Can you work these out from the model? Positions are in its coordinate system, mm. Face numbers are marked on the shaded views. A direction names the side the tool comes from. Coordinates: 2 decimals unless noted, no trailing zeros. Loops run counter-clockwise (first coordinate to the right, second up) from the corner with the lowest first, then second, coordinate; pieces in that order, holes last. Notation, with made-up numbers: (79, 71) -> (135, 71) arc R32 cw to (135, 100) -> close; hole circle Ø3 at (-1, 6). An arc over 180 degrees is marked (long way). Put each result on its own line as item: value. Start each with the question number.
Item 1: If we section it at C-C on x = -34.5: Please give me the cut outline in (y, z).
Item 2: For the marked faces 1 and 2, which set-ups out of +Z, -Z, +X, -X, +Y, -Y let a thin tool reach every point of the face, with its end or its side?
Item 3: If we section it at A-A on z = -15: Please give me the cut outline in (x, y).
Item 4: If we section it at D-D on y = 43.5: Please give me the cut outline in (x, z), plus the area to 3 significant figures.
Item 5: Please list where these lines run through material, in increasing order: L1, parallel to Y at x = -2.95, z = -15; L2, parallel to Z at x = -0.9, y = 32; L3, parallel to X at y = 31, z = -33. Write a range as from..to.
Item 6: Will these pins go through, and if not, where does the flat tip stop? P1, Ø10, axis at x = -24, y = 9.5, coming from the -Z side; P2, Ø12, axis at y = 36.5, z = -29.5, coming from the -X side.
Item 7: If we section it at B-B on y = 52: Please give me the cut outline in (x, z), plus the area to 3 significant figures.
Autodesk Inventor part; units mm, degrees
ref_plane "YZ Plane" through (0, 0, 0) normal (1, 0, 0) x (0, 1, 0)
ref_plane "XZ Plane" through (0, 0, 0) normal (0, 1, 0) x (-1, 0, 0)
ref_plane "XY Plane" through (0, 0, 0) normal (0, 0, 1) x (1, 0, 0)
sketch "スケッチ1" plane through (0, 0, 0) normal (0, 1, 0) x (-1, 0, 0)
  line L0 (0, 0) -> (0, -35)
  line L1 (0, -35) -> (4, -35)
  line L2 (4, -35) -> (4, -4)
  line L3 (4, -4) -> (50, -4)
  line L4 (50, -4) -> (50, 0)
  line L5 (50, 0) -> (0, 0)
  dimension "d0" = 35
  dimension "d1" = 4
  dimension "d2" = 90
  dimension "d3" = 31
  dimension "d4" = 46
extrude "押し出し1" add sketch "スケッチ1" along normal blind 60
sketch "スケッチ2" plane through (-50, 0, 0) normal (0, 0, 1) x (1, 0, 0)
  line L0 (50, 0) -> (50, 60)
  line L1 (0, 0) -> (50, 0)
  point P0 (17.3731, 15.0322)
  dimension "d7" = 32.6269
  dimension "d8" = 15.0322
hole "穴1" at (-32.6269, 15.0322, 0) direction (0, 0, -1) diameter 10 end through all
sketch "スケッチ3" plane through (0, 0, 0) normal (1, 0, 0) x (0, 0, -1)
  line L0 (0, 0) -> (35, 0)
  line L1 (35, 0) -> (35, 60)
  line L2 (0, 0) -> (0, 60)
  line L3 (0, 60) -> (35, 60)
  point P0 (15, 32)
  point P1 (15, 52)
  dimension "d16" = 32
  dimension "d22" = 8
  dimension "d31" = 15
  dimension "d32" = 15
hole "穴2" at (0, 32, -15) at (0, 52, -15) direction (-1, 0, 0) diameter 8 end through all
properties part number "ブレーキ固定アングル"
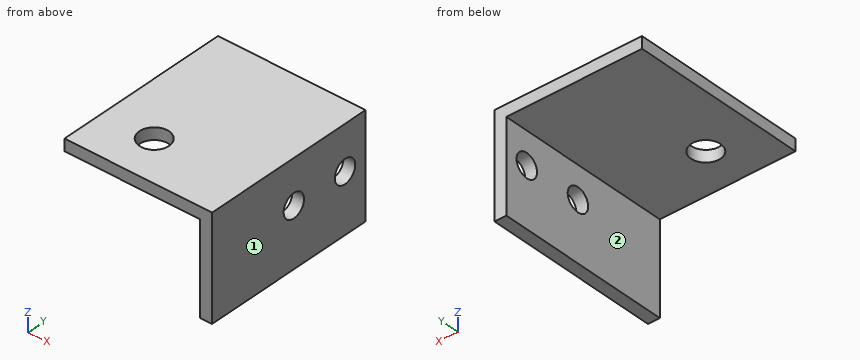
Solutions:
1. outline: (0, -4) -> (10.4, -4) -> (10.4, 0) -> (0, 0) -> close; (19.67, -4) -> (60, -4) -> (60, 0) -> (19.67, 0) -> close
2. face 1: +Z, -Z, +X, +Y, -Y
2. face 2: -Z, -X, +Y, -Y
3. outline: (-4, 0) -> (0, 0) -> (0, 28) -> (-4, 28) -> close; (-4, 36) -> (0, 36) -> (0, 48) -> (-4, 48) -> close; (-4, 56) -> (0, 56) -> (0, 60) -> (-4, 60) -> close
4. outline: (-50, -4) -> (-4, -4) -> (-4, -35) -> (0, -35) -> (0, 0) -> (-50, 0) -> close
4. area: 324 mm^2
5. L1: 0..28, 36..48, 56..60
5. L2: -35..-19, -11..0
5. L3: -4..0
6. P1: z = -4
6. P2: x = -4
7. outline: (-50, -4) -> (-4, -4) -> (-4, -11) -> (0, -11) -> (0, 0) -> (-50, 0) -> close; (-4, -35) -> (0, -35) -> (0, -19) -> (-4, -19) -> close
7. area: 292 mm^2
